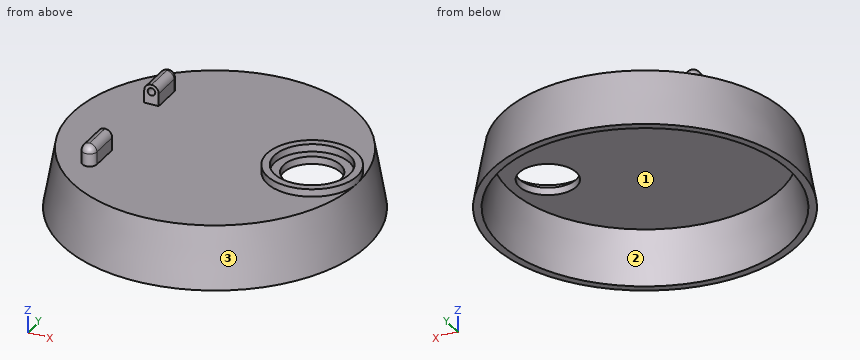
from build123d import *

# Parameters (mm, degrees)
F0_R           = 64.4326190009
F1_DEPTH       = 25.4
F1_TAPER       = 10
F2_T           = -3.175
F3_R           = 19.05
F3_R_2         = 15.875
F4_DEPTH       = 3.175
F3_R_3         = 12.065
F5_DEPTH       = 25.4
F7_DEPTH       = 8.382
F8_R           = 3.048
F9_R           = 1.5875
F10_DEPTH      = 25.4
F10_DEPTH_BACK = 25.4


with BuildPart() as f1:
    # F0 (on Top) → F1 (new body)
    with BuildSketch(Plane.XY):
        Circle(F0_R)
    extrude(amount=F1_DEPTH, taper=F1_TAPER)

    # F2
    f2_openings = [f1.faces().sort_by_distance(p)[0] for p in [
        (0, 0, 0),
    ]]
    offset(amount=F2_T, openings=f2_openings)

    # F3 (on face) → F4 (join)
    with BuildSketch(Plane.XY.offset(25.4)):
        with Locations((40.9039136909, 0)):
            Circle(F3_R)
        with Locations((40.9039136909, 0)):
            Circle(F3_R_2, mode=Mode.SUBTRACT)
    extrude(amount=F4_DEPTH)

    # F3 (on face) → F5 (cut)
    with BuildSketch(Plane.XY.offset(25.4)):
        with Locations((40.9039136909, 0)):
            Circle(F3_R_3)
    extrude(amount=-F5_DEPTH, mode=Mode.SUBTRACT)

    # F6 (on face) → F7 (join)
    with BuildSketch(Plane.XY.offset(25.4)):
        with BuildLine():
            Line((-33.4835186865, -31.5588308226), (-33.4835186865, -19.05))
            Line((-33.4835186865, -19.05), (-39.5865455006, -19.05))
            Line((-39.5865455006, -19.05), (-39.5865455006, -31.5588308226))
            ThreePointArc((-39.5865455006, -31.5588308226), (-36.5350320935, -34.6103442296), (-33.4835186865, -31.5588308226))
        make_face()
        with BuildLine():
            Line((-39.5865455006, 31.5588308226), (-39.5865455006, 19.05))
            Line((-39.5865455006, 19.05), (-33.4835186865, 19.05))
            Line((-33.4835186865, 19.05), (-33.4835186865, 31.5588308226))
            ThreePointArc((-33.4835186865, 31.5588308226), (-36.5350320935, 34.6103442296), (-39.5865455006, 31.5588308226))
        make_face()
    extrude(amount=F7_DEPTH)

    # F8
    f8_edges = [f1.edges().sort_by_distance(p)[0] for p in [
        (-33.483519, -25.304415, 33.782),
        (-39.586546, -25.304415, 33.782),
        (-36.535032, -34.610344, 33.782),
        (-33.483519, 25.304415, 33.782),
    ]]
    fillet(f8_edges, radius=F8_R)

    # F9 (on Front) → F10 (cut, two sides)
    with BuildSketch(Plane.XZ) as f10_sk:
        with Locations((-36.5315186865, 30.734)):
            Circle(F9_R)
    extrude(amount=F10_DEPTH, mode=Mode.SUBTRACT)
    extrude(f10_sk.sketch, amount=-F10_DEPTH_BACK, mode=Mode.SUBTRACT)


solid = f1.part
Part model, mm, in its own coordinate system. Face numbers are marked on the shaded views. Coordinates: 2 decimals unless noted, no trailing zeros. Order: outer loops, then holes, each group sorted by start corner. A loop starts at its lowest first (then second) coordinate and runs counter-clockwise, first axis right, second up. Notation, with made-up numbers: M 71,-11 L 111,-11 A35 cw 111,23 Z; hole C -26,52 d5. An arc over 180 degrees is marked long. Use a Markdown table: item, result.
(1) Flat gauge pins, fed straight in: pin 1 (5 mm diameter, centred on x = -9, y = -23, fed in from +Z); pin 2 (2.5 mm diameter, centred on x = -36.53, z = 30.73, fed in from -Y); pin 3 (5 mm diameter, centred on y = -0.5, z = 28.5, fed in from -X); pin 4 (21.5 mm diameter, centred on x = 40.9, y = 0, fed in from -Z). Where does each tip first touch, or does it go through?
A:
| item | result |
|---|---|
| pin 1 | stops at z = 25.4 |
| pin 2 | stops at y = -34.61 |
| pin 3 | stops at x = 21.85 |
| pin 4 | passes through |
(2) Probe L1, parallel to Z at x = -7, y = -10 (3 decimals); L2, parallel to Y at x = 39.5, z = 10.5; L3, parallel to X at y = -48, z = 20. List the from-to ranges inside material, lowest first.
A:
| item | result |
|---|---|
| L1 | z = 22.225 to 25.4 |
| L2 | y = -48.54 to -44.31, 44.31 to 48.54 |
| L3 | x = -37.49 to -31.99, 31.99 to 37.49 |
(3) Cut at B-B on z = 9.5. Write the cut outline in (x, y).
A:
| item | result |
|---|---|
| outline | C 0,0 d125.52; hole C 0,0 d119.07 |
(4) Cut at A-A on x = 0. Write the cut outline in (y, z) (3 decimals).
A:
| item | result |
|---|---|
| outline | M -64.433,0 L -61.209,0 L -57.29,22.225 L 57.29,22.225 L 61.209,0 L 64.433,0 L 59.954,25.4 L -59.954,25.4 Z |
(5) Pull direction Y, two halves, no side cores. Call the marked faces 1, 2 and 3: released by +Y, released by -Y, zero draft, split by the parting line, or undercut.
A:
| item | result |
|---|---|
| face 1 | undercut |
| face 2 | undercut |
| face 3 | split by the parting line |
